CAD build for the part. Positions are in the model's coordinates, mm. Give positions to 0.01 mm unless a question says otherwise; leave off trailing zeros. Loops run counter-clockwise (first coordinate to the right, second up) from the corner with the lowest first, then second, coordinate; pieces in that order, holes last. Notation, with made-up numbers: (-32.75, 25) - (-25.75, 25) arc R10 ccw to (-25.75, 37) - close; hole circle Ø10 at (27, -6.5). An arc over 180 degrees is marked (long way). Return JSON: item names as keys, results as strings.
from build123d import *

# Parameters (mm, degrees)
F1_DEPTH = 1.5


with BuildPart() as f1:
    # F0 (on Front) → F1 (new body, symmetric)
    with BuildSketch(Plane.XZ):
        Polygon((-60, 15.5), (-98, 15.5), (-98, -3.5), (-101, -3.5), (-101, -9.5), (-98, -9.5), (-98, -15.5), (98, -15.5), (98, -9.5), (101, -9.5), (101, -3.5), (98, -3.5), (98, 15.5), (60, 15.5), (60, 18.5), (40, 18.5), (40, 15.5), (0, 15.5), (-40, 15.5), (-40, 18.5), (-60, 18.5), align=None)
    extrude(amount=F1_DEPTH, both=True)


solid = f1.part
1. Cut at A-A, the plane y = 0.3. Write the cut outline in (x, z), plus the area to 3 significant figures.
Values follow:
{"outline": "(-101, -9.5) - (-98, -9.5) - (-98, -15.5) - (98, -15.5) - (98, -9.5) - (101, -9.5) - (101, -3.5) - (98, -3.5) - (98, 15.5) - (60, 15.5) - (60, 18.5) - (40, 18.5) - (40, 15.5) - (-40, 15.5) - (-40, 18.5) - (-60, 18.5) - (-60, 15.5) - (-98, 15.5) - (-98, -3.5) - (-101, -3.5) - close", "area": "6,230 mm²"}
2. Drop flat-ended pins along their axis: P1, Ø1.5, axis at x = 70.5, y = -0.5, coming from the +Z side; P2, Ø0.9, axis at y = -0.5, z = 3, coming from the +X side; P3, Ø0.9, axis at y = -0.5, z = 1.5, coming from the -X side. Give the stop position or say it passes through.
Values follow:
{"P1": "stops at z = 15.5", "P2": "stops at x = 98", "P3": "stops at x = -98"}
3. Cut at C-C, the plane z = 10. Write the cut outline in (x, y).
Values follow:
{"outline": "(-98, -1.5) - (98, -1.5) - (98, 1.5) - (-98, 1.5) - close"}
4. Cut at B-B, the plane x = 89. Write the cut outline in (y, z).
Values follow:
{"outline": "(-1.5, -15.5) - (1.5, -15.5) - (1.5, 15.5) - (-1.5, 15.5) - close"}
5. Drill centre lines: probe 1 along X at (y, z) = (0, 7); probe 2 along Z at (x, y) = (-3, -0.95). Where is each one in solid material? Low to high.
Values follow:
{"probe 1": "x = -98 to 98", "probe 2": "z = -15.5 to 15.5"}
